from build123d import *

# Parameters (mm, degrees)
BOSS_EXTRUDE1_DEPTH             = 19.05
F_43_0_089_DIAMETER_HOLE1_D     = 2.2606
F_43_0_089_DIAMETER_HOLE1_DEPTH = 25.4
F_43_0_089_DIAMETER_HOLE1_TIP   = 0.679152758
F_43_0_089_DIAMETER_HOLE2_D     = 2.2606
F_43_0_089_DIAMETER_HOLE2_DEPTH = 25.4
F_43_0_089_DIAMETER_HOLE2_TIP   = 0.679152758


with BuildPart() as part:
    # Sketch1 → Boss-Extrude1 (new body)
    with BuildSketch(Plane(origin=(0, 0, 0), x_dir=(0, 0, -1), z_dir=(1, 0, 0))):
        Polygon((0, 0), (0, 12.7), (3.175, 12.7), (3.175, 3.175), (12.7, 3.175), (12.7, 0), align=None)
    extrude(amount=BOSS_EXTRUDE1_DEPTH)

    # #43 (0.089) Diameter Hole1
    with Locations(Plane(origin=(0, 0, -3.175), x_dir=(-1, 0, 0), z_dir=(0, 0, -1))):
        with Locations((-6.35, 7.9375), (-12.7, 7.9375)):
            Hole(F_43_0_089_DIAMETER_HOLE1_D / 2, depth=F_43_0_089_DIAMETER_HOLE1_DEPTH)
            with Locations((0, 0, -(F_43_0_089_DIAMETER_HOLE1_DEPTH + F_43_0_089_DIAMETER_HOLE1_TIP / 2))):  # 118° drill point
                Cone(0, F_43_0_089_DIAMETER_HOLE1_D / 2, F_43_0_089_DIAMETER_HOLE1_TIP, mode=Mode.SUBTRACT)

    # #43 (0.089) Diameter Hole2
    with Locations(Plane(origin=(0, 3.175, 0), x_dir=(1, 0, 0), z_dir=(0, 1, 0))):
        with Locations((6.35, 7.9375), (12.7, 7.9375)):
            Hole(F_43_0_089_DIAMETER_HOLE2_D / 2, depth=F_43_0_089_DIAMETER_HOLE2_DEPTH)
            with Locations((0, 0, -(F_43_0_089_DIAMETER_HOLE2_DEPTH + F_43_0_089_DIAMETER_HOLE2_TIP / 2))):  # 118° drill point
                Cone(0, F_43_0_089_DIAMETER_HOLE2_D / 2, F_43_0_089_DIAMETER_HOLE2_TIP, mode=Mode.SUBTRACT)


solid = part.part
Geometry: final body of the model. Coordinates: model frame, mm. A direction names the side the tool comes from. Coordinates: 2 decimals unless noted, no trailing zeros. Write each loop counter-clockwise with the first axis right and the second up, starting at its lowest first coordinate (ties: lowest second). Pieces come first, ordered by that corner, then holes. Notation, with made-up numbers: (-20, 84.25) - (11, 84.25) arc R36 cw to (11, 123.25) - close; hole circle Ø11 at (61, 59). An arc over 180 degrees is marked (long way). Return JSON: item names as keys, results as strings.
Item 1: Section query A-A (x = 6.35). Output: boundary loops of the cut face in (y, z) (3 decimals), and give its area (3 significant figures).
Completed:
{"outline": "(0, -12.7) - (3.175, -12.7) - (3.175, -9.068) - (0, -9.068) - close; (0, -6.807) - (3.175, -6.807) - (3.175, -3.175) - (6.807, -3.175) - (6.807, 0) - (0, 0) - close; (9.068, -3.175) - (12.7, -3.175) - (12.7, 0) - (9.068, 0) - close", "area": "56.2 mm2"}
Item 2: Pin query (flat end, axial travel): pin 1 Ø1.5 at (x, z) = (5, -10.5) entering from +Y (3 decimals); pin 2 Ø1.5 at (x, y) = (11, 11) entering from -Z (3 decimals). Return the tip coordinate at first contact, or that it passes through.
Completed:
{"pin 1": "stops at y = 3.175", "pin 2": "stops at z = -3.175"}
Item 3: Section query C-C (x = 11). Output: boundary loops of the cut face in (y, z) (3 decimals), and give its area (3 significant figures).
Completed:
{"outline": "(0, -12.7) - (3.175, -12.7) - (3.175, -3.175) - (12.7, -3.175) - (12.7, 0) - (0, 0) - close", "area": "70.6 mm2"}
Item 4: Section query B-B (y = 8.5). Output: boundary loops of the cut face in (x, z) (3 decimals).
Completed:
{"outline": "(0, -3.175) - (5.37, -3.175) - (5.37, 0) - (0, 0) - close; (7.33, -3.175) - (11.72, -3.175) - (11.72, 0) - (7.33, 0) - close; (13.68, -3.175) - (19.05, -3.175) - (19.05, 0) - (13.68, 0) - close"}
Item 5: Section query D-D (y = 6.25). Output: boundary loops of the cut face in (x, z) (3 decimals), and give its area (3 significant figures).
Completed:
{"outline": "(0, -3.175) - (19.05, -3.175) - (19.05, 0) - (0, 0) - close", "area": "60.5 mm2"}
Item 6: Line query: L1, parallel to X at y = 8, z = -1; L2, parallel to Z at x = 6.35, y = 0.75; L3, parallel to Y at x = 13.25, z = -5.75 (3 decimals). Output: solid intervals per line, ascending.
Completed:
{"L1": "x = 0 to 5.22, 7.48 to 11.57, 13.83 to 19.05", "L2": "z = -12.7 to -9.07, -6.81 to 0", "L3": "y = 0 to 3.175"}
Item 7: Pull-direction query (X, two-part tool) for faces 1 (the face through (13.83, 1.57, -7.99)), 2 (the face through (5.272, 1.565, -8.277)), 3 (the face through (0, 4, -2)), 4 (the face through (9, 12.7, -2)); classes: +X half, -X half, draft (parallel to the pull), parting line (faces both ways), or undercut.
Completed:
{"face 1": "undercut", "face 2": "undercut", "face 3": "-X half", "face 4": "draft"}
Item 8: Reachability of faces 5 (the face through (19.05, 4, -2)), 6 (the face through (9, 8, -3.175)) from +Z, -Z, +X, -X, +Y, -Y: full face, straight path, thin tool, end or side. Return the list, or none.
Completed:
{"face 5": "+Z, -Z, +X, +Y, -Y", "face 6": "-Z, +X, -X, +Y"}
